Work out the finished part from the listing and answer in its coordinate system (mm). Face numbers are marked on the shaded views. Round coordinates to 2 decimals unless told otherwise and drop trailing zeros. Loops run counter-clockwise (first coordinate to the right, second up) from the corner with the lowest first, then second, coordinate; pieces in that order, holes last. Notation, with made-up numbers: (66, 48.5) -> (115, 48.5) arc R22 cw to (115, 86.5) -> close; hole circle Ø1 at (-24.5, -26.5). An arc over 180 degrees is marked (long way). Use one line per item in the form item = value.
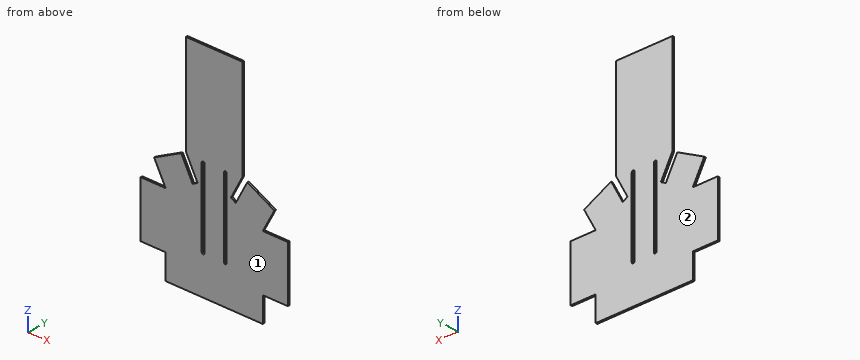
```python
from build123d import *

# Parameters (mm, degrees)
BASE_DEPTH          = 3.175
SKETCH2_W           = 175
SKETCH2_H           = 45
BOSS_EXTRUDE2_DEPTH = 3.175
SKETCH3_W           = 45
SKETCH3_H           = 100
BOSS_EXTRUDE3_DEPTH = 3.175
CUT_EXTRUDE1_DEPTH  = 375.254366207


with BuildPart() as part:
    # Sketch1 → Base (new body)
    with BuildSketch(Plane(origin=(0, 0, 0), x_dir=(1, 0, 0), z_dir=(0, 1, 0))):
        Polygon((87.5, 0), (-87.5, 0), (-87.5, -100), (-30, -130), (-30, -350), (30, -350), (30, -130), (87.5, -100), align=None)
    extrude(amount=BASE_DEPTH)

    # Sketch2 → Boss-Extrude2 (add)
    with BuildSketch(Plane(origin=(0, 0, 0), x_dir=(1, 0, 0), z_dir=(0, 1, 0))):
        with Locations((0, 22.5)):
            Rectangle(SKETCH2_W, SKETCH2_H)
        Polygon((-108.315470301, -139.896318077), (-87.5, -100), (-38.733948559, -125.03895229), (-59.553303762, -165.337448446), align=None)
        Polygon((108.315470301, -139.896318077), (59.553303762, -165.337448446), (38.733948559, -125.03895229), (87.5, -100), align=None)
        Polygon((-30, -130), (-50.819355203, -170.298496155), (-50.819355203, -350), (-30, -350), align=None)
        Polygon((50.819355203, -170.298496155), (50.819355203, -350), (30, -350), (30, -130), align=None)
    extrude(amount=BOSS_EXTRUDE2_DEPTH)

    # Sketch3 → Boss-Extrude3 (add)
    with BuildSketch(Plane(origin=(0, 0, 0), x_dir=(1, 0, 0), z_dir=(0, 1, 0))):
        with Locations((-110, -50)):
            Rectangle(SKETCH3_W, SKETCH3_H)
        with Locations((110, -50)):
            Rectangle(SKETCH3_W, SKETCH3_H)
    extrude(amount=BOSS_EXTRUDE3_DEPTH)

    # Sketch4 → Cut-Extrude1 (cut, through all)
    with BuildSketch(Plane(origin=(0, 3.175, 0), x_dir=(1, 0, 0), z_dir=(0, 1, 0))):
        with BuildLine():
            Line((-17.5, -25), (-17.5, -165))
            ThreePointArc((-17.5, -165), (-20, -167.5), (-22.5, -165))
            Line((-22.5, -165), (-22.5, -25))
            ThreePointArc((-22.5, -25), (-20, -22.5), (-17.5, -25))
        make_face()
        with BuildLine():
            Line((17.5, -25), (17.5, -165))
            ThreePointArc((17.5, -165), (20, -167.5), (22.5, -165))
            Line((22.5, -165), (22.5, -25))
            ThreePointArc((22.5, -25), (20, -22.5), (17.5, -25))
        make_face()
    extrude(amount=-CUT_EXTRUDE1_DEPTH, mode=Mode.SUBTRACT)


solid = part.part
```
(1) Find section C-C, the plane x = 73.5. Write down the section's boundary in (y, z) (3 decimals).
Completed:
outline = (0, -45) -> (3.175, -45) -> (3.175, 158.061) -> (0, 158.061) -> close
(2) Consider L1, parallel to X at y = 1.4, z = 34; L2, parallel to X at y = 2.75, z = 139; L3, parallel to X at y = 1.35, z = 166. Determine where each line is inside the solid, lowest interval first.
Completed:
L1 = -132.5 to -22.5, -17.5 to 17.5, 22.5 to 132.5
L2 = -107.85 to -45.95, -34.65 to -22.5, -17.5 to 17.5, 22.5 to 34.65, 45.95 to 107.85
L3 = -48.6 to -22.29, -17.71 to 17.71, 22.29 to 48.6
(3) Find section D-D, the plane z = 309.5. Write down the section's boundary in (x, y) (3 decimals).
Completed:
outline = (-50.819, 0) -> (50.819, 0) -> (50.819, 3.175) -> (-50.819, 3.175) -> close
(4) Find section B-B, the plane z = 61.5. Write down the section's boundary in (x, y) (3 decimals), then the cut area to 3 significant figures.
Completed:
outline = (-132.5, 0) -> (-22.5, 0) -> (-22.5, 3.175) -> (-132.5, 3.175) -> close; (-17.5, 0) -> (17.5, 0) -> (17.5, 3.175) -> (-17.5, 3.175) -> close; (22.5, 0) -> (132.5, 0) -> (132.5, 3.175) -> (22.5, 3.175) -> close
area = 810 mm2
(5) Find section A-A, the plane y = 1.8. State how many separate pieces and enclosed holes the cut face has, then the cut area to 3 significant figures.
Completed:
separate_pieces = 1
enclosed_holes = 2
area = 62,900 mm2
(6) For a pull along Y with two mould halves and no side action, classify the marked faces 1 and 2 as +Y half, -Y half, draft (parallel to the pull), parting line (faces both ways), or undercut.
Completed:
face_1 = -Y half
face_2 = +Y half
(7) Given P1, Ø1, axis at y = 2, z = -12.5, coming from the -X side; P2, Ø4, axis at x = 105, z = 128.5, coming from the -Y side; P3, Ø1.6, axis at y = 2, z = 299, coming from the +X side; P4, Ø1, axis at x = 108.5, y = 1, coming from the -Z side, each flat-ended and moving along its own axis, determine where each tip first touches the part or whether it passes through.
Completed:
P1 = -87.5
P2 = through
P3 = 50.82
P4 = 0
